```python
from build123d import *

# Parameters (mm, degrees)
SKETCH1_R           = 1.5
SKETCH1_R_2         = 2.5
BOSS_EXTRUDE1_DEPTH = 3.175
FILLET1_R           = 3


with BuildPart() as part:
    # Sketch1 → Boss-Extrude1 (new body)
    with BuildSketch(Plane(origin=(0, 0, 0), x_dir=(1, 0, 0), z_dir=(0, 1, 0))):
        with BuildLine():
            Line((0, -14), (0, 14))
            Line((0, 14), (20, 14))
            Line((20, 14), (39.625823576, 21.230243699))
            ThreePointArc((39.625823576, 21.230243699), (46.990090369, 20.282681475), (50.425, 13.7))
            Line((50.425, 13.7), (50.425, 6))
            Line((50.425, 6), (68, 6))
            Line((68, 6), (68, -6))
            Line((68, -6), (50.425, -6))
            Line((50.425, -6), (50.425, -13.7))
            ThreePointArc((50.425, -13.7), (46.990090369, -20.282681475), (39.625823576, -21.230243699))
            Line((39.625823576, -21.230243699), (20, -14))
            Line((20, -14), (0, -14))
        make_face()
        with Locations((2.5, 8)):
            Circle(SKETCH1_R, mode=Mode.SUBTRACT)
        with Locations((17.5, 8)):
            Circle(SKETCH1_R, mode=Mode.SUBTRACT)
        with Locations((17.5, -8)):
            Circle(SKETCH1_R, mode=Mode.SUBTRACT)
        with Locations((2.5, -8)):
            Circle(SKETCH1_R, mode=Mode.SUBTRACT)
        with Locations((42.4, 13.7)):
            Circle(SKETCH1_R_2, mode=Mode.SUBTRACT)
        with Locations((42.4, -13.7)):
            Circle(SKETCH1_R_2, mode=Mode.SUBTRACT)
        with Locations((36, 0)):
            Circle(SKETCH1_R, mode=Mode.SUBTRACT)
        with Locations((61, 0)):
            Circle(SKETCH1_R, mode=Mode.SUBTRACT)
    extrude(amount=BOSS_EXTRUDE1_DEPTH)

    # Fillet1
    fillet1_edges = [part.edges().sort_by_distance(p)[0] for p in [
        (0, 1.5875, 14),
        (0, 1.5875, -14),
        (20, 1.5875, -14),
        (68, 1.5875, -6),
        (68, 1.5875, 6),
        (20, 1.5875, 14),
    ]]
    fillet(fillet1_edges, radius=FILLET1_R)


solid = part.part
```
Geometry check sheet. Reference: the model listing, model coordinates, mm. A direction names the side the tool comes from. Give positions to 0.01 mm unless a question says otherwise; leave off trailing zeros. Write each loop counter-clockwise with the first axis right and the second up, starting at its lowest first coordinate (ties: lowest second). Pieces come first, ordered by that corner, then holes.
1) Access from +Z, -Z, +X, -X, +Y, -Y to the whole of each face (thin tool, end or side, straight path). Record for faces 1 (the flat face through (50.425, 2, 10)), 2 (the cylindrical face through (16, 2, 8)), 3 (the flat face through (11, 2, 14)), 4 (the flat face through (50.425, 2, -10)).
2) Material ranges on L1, parallel to X at y = 1.6, z = 0; L2, parallel to X at y = 0.95, z = 8 (3 decimals); L3, parallel to Z at x = 61, y = 1.1, recorded low to high.
3) Section check B-B, the plane x = 61. Record the boundary of the cut face in (y, z) (3 decimals).
4) Release check for a two-part mould opening along X. For faces 5 (the cylindrical face through (2.175, 1.565, 9.464)), 6 (the flat face through (11, 2, -14)), 7 (the flat face through (68, 2, 0)) record: pulls with the +X half, pulls with the -X half, needs draft (parallel to the pull), parting line crosses it, or undercut.
5) Section check D-D, the plane z = -12.5. Record the boundary of the cut face in (x, y) (3 decimals).
6) Section check A-A, the plane z = 8. Record the boundary of the cut face in (x, y) (3 decimals), and give its area (3 significant figures).
7) Section check C-C, the plane y = 0.7. State how many separate pieces and enclosed holes the cut face has, and give its area (3 significant figures).
8) Gauge pin test, flat ends, axial feed: pin 1 (4 mm diameter, centred on x = 42.4, z = -13.7, fed in from +Y); pin 2 (1.6 mm diameter, centred on x = 57.5, y = 1, fed in from -Z); pin 3 (1.6 mm diameter, centred on y = 2, z = 11, fed in from +X) (3 decimals); pin 4 (1 mm diameter, centred on x = 8, y = 2, fed in from -Z). Record the tip position at first contact, or that the pin passes through.
Computed:
1. face 1: +Z, +X, +Y, -Y
1. face 2: +Y, -Y
1. face 3: +Z, -X, +Y, -Y
1. face 4: -Z, +X, +Y, -Y
2. L1: x = 0 to 34.5, 37.5 to 59.5, 62.5 to 68
2. L2: x = 0 to 1, 4 to 16, 19 to 50.425
2. L3: z = -6 to -1.5, 1.5 to 6
3. outline: (0, -6) - (3.175, -6) - (3.175, -1.5) - (0, -1.5) - close; (0, 1.5) - (3.175, 1.5) - (3.175, 6) - (0, 6) - close
4. face 5: undercut
4. face 6: needs draft
4. face 7: pulls with the +X half
5. outline: (0.402, 0) - (40.207, 0) - (40.207, 3.175) - (0.402, 3.175) - close; (44.593, 0) - (50.425, 0) - (50.425, 3.175) - (44.593, 3.175) - close
6. outline: (0, 0) - (1, 0) - (1, 3.175) - (0, 3.175) - close; (4, 0) - (16, 0) - (16, 3.175) - (4, 3.175) - close; (19, 0) - (50.425, 0) - (50.425, 3.175) - (19, 3.175) - close
6. area: 141 mm2
7. separate pieces: 1
7. enclosed holes: 8
7. area: 1,810 mm2
8. pin 1: passes through
8. pin 2: stops at z = -6
8. pin 3: stops at x = 50.425
8. pin 4: stops at z = -14
